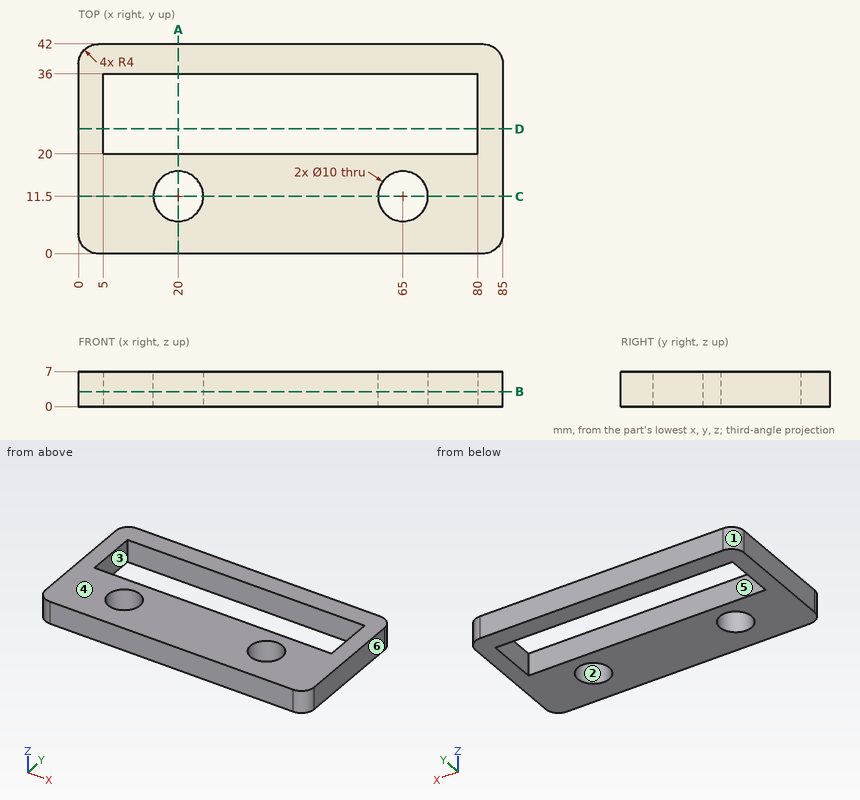
The drawing under review shows one solid part. Ordinate dimensions are in mm from its lowest x, y, z. A direction names the side the tool comes from. Round coordinates to 2 decimals unless told otherwise and drop trailing zeros. Write each loop counter-clockwise with the first axis right and the second up, starting at its lowest first coordinate (ties: lowest second). Pieces come first, ordered by that corner, then holes. Notation, with made-up numbers: (30, 62) -> (41, 62) arc R9 cw to (41, 71) -> close; hole circle Ø11 at (-8, 87.25). An arc over 180 degrees is marked (long way). Put each result on its own line as item: value.
Q1. Consider section D-D on y = 25. State the section outline as (x, z) points.
Determined:
outline: (0, 0) -> (5, 0) -> (5, 7) -> (0, 7) -> close; (80, 0) -> (85, 0) -> (85, 7) -> (80, 7) -> close
Q2. Consider section C-C on y = 11.5. State the section outline as (x, z) points, and give its area (3 significant figures).
Determined:
outline: (0, 0) -> (15, 0) -> (15, 7) -> (0, 7) -> close; (25, 0) -> (60, 0) -> (60, 7) -> (25, 7) -> close; (70, 0) -> (85, 0) -> (85, 7) -> (70, 7) -> close
area: 455 mm^2
Q3. To check wall thickness, follow L1, parallel to Y at x = 65, z = 4.25; L2, parallel to X at y = 31.5, z = 5.5; L3, parallel to Y at x = 34.5, z = 1.75. State the ranges of each line that lie inside material, in increasing order. Write a range as [from, to].
Determined:
L1: y = [0, 6.5], [16.5, 20], [36, 42]
L2: x = [0, 5], [80, 85]
L3: y = [0, 20], [36, 42]
Q4. Consider section B-B on z = 3. State the section outline as (x, y) points.
Determined:
outline: (0, 4) arc R4 ccw to (4, 0) -> (81, 0) arc R4 ccw to (85, 4) -> (85, 38) arc R4 ccw to (81, 42) -> (4, 42) arc R4 ccw to (0, 38) -> close; hole (5, 20) -> (80, 20) -> (80, 36) -> (5, 36) -> close; hole circle Ø10 at (20, 11.5); hole circle Ø10 at (65, 11.5)
Q5. Consider section A-A on x = 20. State the section outline as (y, z) points, and give its area (3 significant figures).
Determined:
outline: (0, 0) -> (6.5, 0) -> (6.5, 7) -> (0, 7) -> close; (16.5, 0) -> (20, 0) -> (20, 7) -> (16.5, 7) -> close; (36, 0) -> (42, 0) -> (42, 7) -> (36, 7) -> close
area: 112 mm^2
Q6. The part is to be moulded in two halves that separate along X. For the marked faces 1, 2, 3 and 4, say which applies: released by +X, released by -X, zero draft, split by the parting line, or undercut.
Determined:
face 1: released by -X
face 2: undercut
face 3: undercut
face 4: zero draft
Q7. Machinability: for the marked faces 5 and 6, which of the approach directions +Z, -Z, +X, -X, +Y, -Y give a long, thin tool a straight path to every point of the face, cutting with its end or side? Answer none if there is none.
Determined:
face 5: +Z, -Z
face 6: +Z, -Z, +X, +Y, -Y
